The listing builds one solid part. Answer for the finished solid, in the listing's coordinates (mm). A direction names the side the tool comes from. Coordinates: 2 decimals unless noted, no trailing zeros. Loops run counter-clockwise (first coordinate to the right, second up) from the corner with the lowest first, then second, coordinate; pieces in that order, holes last. Notation, with made-up numbers: (77, -16.5) -> (131, -16.5) arc R17 cw to (131, 0.5) -> close; hole circle Ø8 at (-12.75, 28). An arc over 180 degrees is marked (long way). Answer in a Markdown table with one row per item.
Autodesk Inventor part; units mm, degrees
ref_plane "Work Plane1" through (0, 7.5, 0) normal (0, 1, 0) x (1, 0, 0)
ref_plane "Work Plane2" through (0, 5, 0) normal (0, -1, 0) x (1, 0, 0)
ref_plane "Work Plane3" through (7.5, 0, 0) normal (1, 0, 0) x (0, 1, 0)
sketch "Sketch1" plane through (0, 0, 0) normal (0, 1, 0) x (-1, 0, 0)
  circle A0 centre (0, 0) radius 5
  circle A1 centre (0, 0) radius 7.5
  dimension "d0" = 10
  dimension "d1" = 15
extrude "Extrusion1" add sketch "Sketch1" along normal blind 10
ref_plane "Work Plane1" through (0, 7.5, 0) normal (0, 1, 0) x (1, 0, 0)
sketch "Sketch2" plane through (0, 7.5, 0) normal (0, 1, 0) x (1, 0, 0)
  line L0 (-5, 5.5902) -> (-5, 15)
  line L1 (-5, 15) -> (5, 15)
  line L2 (5, 15) -> (5, 5.5902)
  circle A0 centre (0, 0) radius 7.5
  circle A1 centre (0, 0) radius 7.5
  dimension "d5" = 10
  dimension "d6" = 5
  dimension "d7" = 15
extrude "Extrusion2" add sketch "Sketch2" along normal blind 2 contours L0 L1 L2 A0
ref_plane "Work Plane2" through (0, 5, 0) normal (0, -1, 0) x (1, 0, 0)
sketch "Sketch4" plane through (0, 7.5, 0) normal (0, -1, 0) x (1, 0, 0)
  circle A0 centre (0, -30) radius 10
  line L0 (5, -5.5902) -> (5, -15)
  line L1 (-5, -15) -> (-5, -5.5902)
  line L2 (-5, -5.5902) -> (-9.7784, -27.9062)
  line L3 (5, -5.5902) -> (9.7784, -27.9062)
  line L4 (5, -15) -> (-5, -15)
  point P0 (0, 0)
  dimension "d11" = 20
  dimension "d26" = 30
sketch "Sketch5" plane through (0, 10, 0) normal (0, 1, 0) x (1, 0, 0)
  line L0 (0, 0) -> (-8, -8)
  line L1 (-8, -8) -> (8, -8)
  line L2 (8, -8) -> (0, 0)
  line L3 (-13.7421, 0) -> (14.2579, 0)
  dimension "d12" = 8
  dimension "d13" = 45
  dimension "d14" = 45
extrude "Extrusion3" cut sketch "Sketch5" against normal blind 10
ref_plane "Work Plane3" through (7.5, 0, 0) normal (1, 0, 0) x (0, 1, 0)
sketch "Sketch6" plane through (7.5, 0, 0) normal (1, 0, 0) x (0, 1, 0)
  point P0 (0, 0)
  point P1 (5, 0)
  dimension "d18" = 5
hole "Hole1" at (7.5, 5, 0) direction (-1, 0, 0) diameter 2.459 end through all
extrude "Extrusion4" add sketch "Sketch4" against normal blind 2
ref_plane "Work Plane5" through (0, 5, 0) normal (0, -1, 0) x (1, 0, 0)
mirror "Mirror2" about plane through (0, 5, 0) normal (0, -1, 0) of "Extrusion2", "Extrusion4"
sketch "Sketch7" plane through (0, 9.5, 0) normal (0, 1, 0) x (1, 0, 0)
  arc A0 (9.7784, 27.9062) -> (-9.7784, 27.9062) centre (0, 30) ccw
  point P0 (0, 0)
hole "Hole2" at (0, 9.5, -30) direction (0, -1, 0) diameter 8.376 end through all
properties part number "KEP_BUT" material "Nickel-Copper Alloy 400"
Item 1: A cutting plane is placed at D-D, the plane x = 0. Determine the outline of the cut face in (y, z).
Findings below:
| item | result |
|---|---|
| outline | (0, -7.5) -> (0.5, -7.5) -> (0.5, -25.81) -> (2.5, -25.81) -> (2.5, -7.5) -> (7.5, -7.5) -> (7.5, -25.81) -> (9.5, -25.81) -> (9.5, -7.5) -> (10, -7.5) -> (10, -5) -> (0, -5) -> close; (0.5, -40) -> (2.5, -40) -> (2.5, -34.19) -> (0.5, -34.19) -> close; (7.5, -40) -> (9.5, -40) -> (9.5, -34.19) -> (7.5, -34.19) -> close |
Item 2: Flat-ended cylindrical pins translate along their axes: pin 1 Ø4 at (x, z) = (-7.5, -21.5) entering from +Y; pin 2 Ø2 at (y, z) = (5, 0) entering from +X; pin 3 Ø1.5 at (y, z) = (9, -20) entering from -X; pin 4 Ø3 at (x, y) = (-5.5, 7.5) entering from +Z. Find the tip coordinate at first contact, or state that the pin passes through.
Findings below:
| item | result |
|---|---|
| pin 1 | stops at y = 9.5 |
| pin 2 | passes through |
| pin 3 | stops at x = -8.25 |
| pin 4 | stops at z = 5.3 |
Item 3: Find the intervals of material crossed by probe 1 along Y at (x, z) = (-7.5, -33); probe 2 along Z at (x, y) = (0, 1.6); probe 3 along Y at (x, z) = (-5.9, 0), in increasing order.
Findings below:
| item | result |
|---|---|
| probe 1 | y = 0.5 to 2.5, 7.5 to 9.5 |
| probe 2 | z = -40 to -34.19, -25.81 to -5 |
| probe 3 | y = 0 to 3.77, 6.23 to 10 |
Item 4: A cutting plane is placed at B-B, the plane x = -6.5. Determine the outline of the cut face in (y, z), plus the area to 3 significant figures.
Findings below:
| item | result |
|---|---|
| outline | (0, -3.74) -> (10, -3.74) -> (10, 3.74) -> (0, 3.74) -> close; (0.5, -37.6) -> (2.5, -37.6) -> (2.5, -12.6) -> (0.5, -12.6) -> close; (7.5, -37.6) -> (9.5, -37.6) -> (9.5, -12.6) -> (7.5, -12.6) -> close; hole circle Ø2.46 at (5, 0) |
| area | 170 mm2 |
Item 5: A cutting plane is placed at A-A, the plane z = -30. Determine the outline of the cut face in (x, y).
Findings below:
| item | result |
|---|---|
| outline | (-10, 0.5) -> (-4.19, 0.5) -> (-4.19, 2.5) -> (-10, 2.5) -> close; (-10, 7.5) -> (-4.19, 7.5) -> (-4.19, 9.5) -> (-10, 9.5) -> close; (4.19, 0.5) -> (10, 0.5) -> (10, 2.5) -> (4.19, 2.5) -> close; (4.19, 7.5) -> (10, 7.5) -> (10, 9.5) -> (4.19, 9.5) -> close |
Item 6: A tool of negligible diameter and unlimited length cuts with its end or side. For faces 4 (the face through (4, 5, 4)), 5 (the face through (0, 5, -5)), 6 (the face through (-7.356, 8.486, -16.592)), 7 (the face through (7.42, 1.51, -16.9)), 8 (the face through (0.1, 0, -5.3)), from which of +Z, -Z, +X, -X, +Y, -Y can it reach the whole face along a straight path? Write none if from no direction.
Findings below:
| item | result |
|---|---|
| face 4 | +Z, +Y, -Y |
| face 5 | +Y, -Y |
| face 6 | -X, +Y, -Y |
| face 7 | +X, +Y, -Y |
| face 8 | +Z, -Z, +X, -X, -Y |
Item 7: Determine the mould class of faces 1 (the face through (0.1, 10, -5.3)), 2 (the face through (-0.247, 4.93, -7.496)), 3 (the face through (-4, 5, 4)) for opening direction Z: +Z half, -Z half, draft (parallel to the pull), parting line (faces both ways), or undercut.
Findings below:
| item | result |
|---|---|
| face 1 | draft |
| face 2 | undercut |
| face 3 | +Z half |
Item 8: A cutting plane is placed at C-C, the plane y = 8.25. Determine the outline of the cut face in (x, z).
Findings below:
| item | result |
|---|---|
| outline | (-9.78, -27.91) arc R10 ccw (long way) to (9.78, -27.91) -> (5, -5.59) arc R7.5 ccw to (5.3, 5.3) -> (3.54, 3.54) arc R5 cw (long way) to (-3.54, 3.54) -> (-5.3, 5.3) arc R7.5 ccw to (-5, -5.59) -> close; hole circle Ø8.38 at (0, -30) |
